The listing builds one solid part. Answer for the finished solid, in the listing's coordinates (mm). A direction names the side the tool comes from. Give positions to 0.01 mm unless a question says otherwise; leave off trailing zeros. Write each loop counter-clockwise with the first axis right and the second up, starting at its lowest first coordinate (ties: lowest second). Pieces come first, ordered by that corner, then holes. Notation, with made-up numbers: M 67.5,19.5 L 121.5,19.5 A16 ccw 121.5,37.5 Z; hole C 63.5,28 d7. An arc over 180 degrees is marked long. Return JSON: item names as keys, results as strings.
from build123d import *

# Parameters (mm, degrees)
CHAFL_N2_SIZE         = 0.3
CHAFL_N2_SIZE2        = 0.212132034
CHAFL_N3_SIZE         = 0.3
CORTAR_EXTRUIR2_DEPTH = 1


with BuildPart() as part:
    # Croquis1 → Revolución1 (revolve)
    with BuildSketch(Plane.XY, mode=Mode.PRIVATE) as revoluci_n1_sk:
        Polygon((0, 0), (3.2, 0), (1.5, -1.7), (1.5, -12), (0, -12), align=None)
    revolve(revoluci_n1_sk.sketch.rotate(Axis((0, 0, 0), (0, -1, 0)), 90), axis=Axis((0, 0, 0), (0, -1, 0)))

    # Chaflán2
    chafl_n2_edges = [part.edges().sort_by_distance(p)[0] for p in [
        (0, 0, -3.2),
    ]]
    chafl_n2_side = [part.faces().sort_by_distance(p)[0] for p in [
        (0, -0.85, -2.35),
    ]]
    chamfer(chafl_n2_edges, length=CHAFL_N2_SIZE, length2=CHAFL_N2_SIZE2, reference=chafl_n2_side[0])

    # Chaflán3
    chafl_n3_edges = [part.edges().sort_by_distance(p)[0] for p in [
        (0, -12, -1.5),
    ]]
    chamfer(chafl_n3_edges, length=CHAFL_N3_SIZE)

    # Croquis3 → Cortar-Extruir2 (cut)
    with BuildSketch(Plane(origin=(0, 0, 0), x_dir=(1, 0, 0), z_dir=(0, 1, 0))):
        Polygon((-0.721687836, 1.25), (-1.443375673, 0), (-0.721687836, -1.25), (0.721687836, -1.25), (1.443375673, 0), (0.721687836, 1.25), align=None)
    extrude(amount=-CORTAR_EXTRUIR2_DEPTH, mode=Mode.SUBTRACT)


solid = part.part
Item 1: Which of the six approach directions +Z, -Z, +X, -X, +Y, -Y give full straight-line access (tool end or side, diameter ignored) to faces 4 (the flat face through (0, -12, 0)), 5 (the flat face through (0, -0.5, -1.25))?
Geometry results:
{"face 4": "+Z, -Z, +X, -X, -Y", "face 5": "+Y"}
Item 2: Find the intervals of material crossed by line 1 (Y direction, x = 0.95, z = -0.45); line 2 (Z direction, x = -0.9, y = -1.5); line 3 (X direction, y = -8.5, z = -1), in increasing order.
Geometry results:
{"line 1": "y = -12 to -1", "line 2": "z = -1.44 to 1.44", "line 3": "x = -1.12 to 1.12"}
Item 3: A cutting plane is placed at A-A, the plane y = -2.5. Write down the section's boundary in (x, z).
Geometry results:
{"outline": "C 0,0 d3"}
Item 4: Given pin 1 Ø2 at (y, z) = (-2.5, -0.5) entering from +X; pin 2 Ø0.5 at (x, y) = (0, -0.5) entering from +Z; pin 3 Ø1 at (x, y) = (-1.5, -9) entering from -Z, each flat-ended and moving along its own axis, determine where each tip first touches the part or whether it passes through.
Geometry results:
{"pin 1": "stops at x = 1.65", "pin 2": "stops at z = 2.95", "pin 3": "stops at z = -1.12"}
Item 5: Determine the mould class of faces 1 (the flat face through (1.08, -0.49, 0.63)), 2 (the cylindrical face through (-0.45, -6.77, 1.43)), 3 (the flat face through (1.3, 0, -0.6)) for opening direction X: +X half, -X half, draft (parallel to the pull), parting line (faces both ways), or undercut.
Geometry results:
{"face 1": "undercut", "face 2": "parting line", "face 3": "draft"}
